from build123d import *

# Parameters (mm, degrees)
SKETCH1_W           = 130
SKETCH1_H           = 160
BOSS_EXTRUDE1_DEPTH = 3.175
SKETCH2_W           = 3.175
SKETCH2_H           = 20
SKETCH2_W_2         = 15
SKETCH2_H_2         = 3.175
SKETCH2_W_3         = 20
CUT_EXTRUDE1_DEPTH  = 3.175


with BuildPart() as part:
    # Sketch1 → Boss-Extrude1 (new body)
    with BuildSketch(Plane.XY):
        with Locations((-10.981871877, 76.825)):
            Rectangle(SKETCH1_W, SKETCH1_H)
    extrude(amount=-BOSS_EXTRUDE1_DEPTH)

    # Sketch2 → Cut-Extrude1 (cut)
    with BuildSketch(Plane.XY):
        with Locations((-74.394371877, 56.825)):
            Rectangle(SKETCH2_W, SKETCH2_H)
        with Locations((-74.394371877, 96.825)):
            Rectangle(SKETCH2_W, SKETCH2_H)
        with Locations((-74.394371877, 136.825)):
            Rectangle(SKETCH2_W, SKETCH2_H)
        with Locations((-68.481871877, 155.2375)):
            Rectangle(SKETCH2_W_2, SKETCH2_H_2)
        with Locations((-30.981871877, 155.2375)):
            Rectangle(SKETCH2_W_3, SKETCH2_H_2)
        with Locations((9.018128123, 155.2375)):
            Rectangle(SKETCH2_W_3, SKETCH2_H_2)
        with Locations((46.518128123, 155.2375)):
            Rectangle(SKETCH2_W_2, SKETCH2_H_2)
        with Locations((52.430628123, 136.825)):
            Rectangle(SKETCH2_W, SKETCH2_H)
        with Locations((52.430628123, 96.825)):
            Rectangle(SKETCH2_W, SKETCH2_H)
        with Locations((52.430628123, 56.825)):
            Rectangle(SKETCH2_W, SKETCH2_H)
        with Locations((52.430628123, 16.825)):
            Rectangle(SKETCH2_W, SKETCH2_H)
        with Locations((46.518128123, -1.5875)):
            Rectangle(SKETCH2_W_2, SKETCH2_H_2)
        with Locations((9.018128123, -1.5875)):
            Rectangle(SKETCH2_W_3, SKETCH2_H_2)
        with Locations((-30.981871877, -1.5875)):
            Rectangle(SKETCH2_W_3, SKETCH2_H_2)
        with Locations((-74.394371877, 16.825)):
            Rectangle(SKETCH2_W, SKETCH2_H)
        with Locations((-68.481871877, -1.5875)):
            Rectangle(SKETCH2_W_2, SKETCH2_H_2)
    extrude(amount=-CUT_EXTRUDE1_DEPTH, mode=Mode.SUBTRACT)


solid = part.part
For this review, take the finished solid that the model builds, in its own axes (mm). A direction names the side the tool comes from. Give positions to 0.01 mm unless a question says otherwise; leave off trailing zeros. Loops run counter-clockwise (first coordinate to the right, second up) from the corner with the lowest first, then second, coordinate; pieces in that order, holes last. Notation, with made-up numbers: (21, 70.25) -> (44, 70.25) arc R17 cw to (44, 98.25) -> close; hole circle Ø7 at (69.5, 41). An arc over 180 degrees is marked (long way). One line per question, with ' | ' between items.
1) The part is to be moulded in two halves that separate along X. For faces 1 (the flat face through (52, 46.825, -2)), 2 (the flat face through (50.843, 97, -2)), 3 (the flat face through (-20.982, -2, -2)), say which applies: +X half, -X half, draft (parallel to the pull), parting line (faces both ways), or undercut.
Resolved:
face 1: draft | face 2: +X half | face 3: undercut
2) We need section B-B (x = -28). Write out the cut boundary in (y, z) (3 decimals), plus the area to 3 significant figures.
Resolved:
outline: (0, -3.175) -> (153.65, -3.175) -> (153.65, 0) -> (0, 0) -> close | area: 488 mm2
3) We need section A-A (y = 51). Write out the cut boundary in (x, z) (3 decimals).
Resolved:
outline: (-72.807, -3.175) -> (50.843, -3.175) -> (50.843, 0) -> (-72.807, 0) -> close
4) For faces 4 (the flat face through (39.018, -2, -2)), 5 (the flat face through (-74, 126.825, -2)), 6 (the flat face through (-0.982, 155, -2)), list the 3-axis set-ups (+Z, -Z, +X, -X, +Y, -Y) from which the entire face can be reached by the end or side of a thin tool; tool diameter is ignored.
Resolved:
face 4: +Z, -Z, +X, -Y | face 5: +Z, -Z, -X | face 6: +Z, -Z, +Y
5) Insertion check: pin 1 Ø1 at (y, z) = (97, -1) entering from +X; pin 2 Ø1 at (x, z) = (53, -2.5) entering from -Y; pin 3 Ø6 at (x, y) = (5, 42) entering from +Z; pin 4 Ø1 at (x, z) = (-68.5, -1) entering from +Y. Each pin has a flat end and moves straight along its axis. Give the tip position at first contact, or say it passes through.
Resolved:
pin 1: stops at x = 50.84 | pin 2: stops at y = 0 | pin 3: stops at z = 0 | pin 4: stops at y = 153.65
6) To check wall thickness, follow probe 1 along X at (y, z) = (91, -1.8); probe 2 along Y at (x, z) = (-22.5, -1). State the ranges of each line that lie inside material, in increasing order.
Resolved:
probe 1: x = -72.81 to 50.84 | probe 2: y = 0 to 153.65
